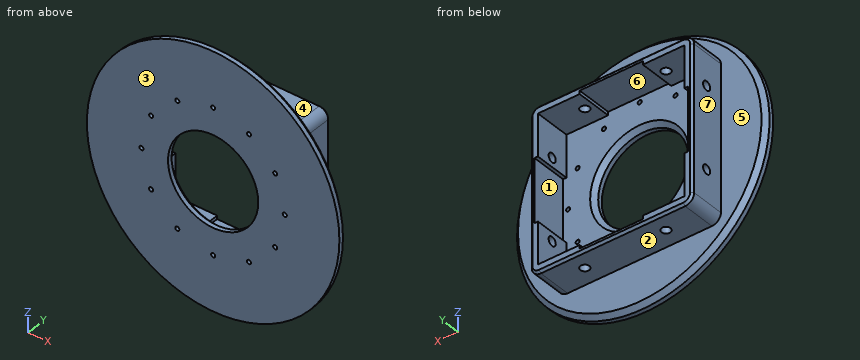
```python
from build123d import *

# Parameters (mm, degrees)
SKETCH1_R               = 88.9
SKETCH1_W               = 114.3
SKETCH1_H               = 114.3
BOSS_EXTRUDE1_DEPTH     = 6.35
SKETCH1_R_2             = 1.4351
SKETCH1_R_3             = 31.75
BOSS_EXTRUDE1_2_DEPTH   = 6.35
SKETCH1_3_W             = 114.3
SKETCH1_3_H             = 114.3
BOSS_EXTRUDE2_DEPTH     = 31.75
SKETCH3_R               = 3.175
CUT_EXTRUDE1_DEPTH      = 89.9
CUT_EXTRUDE1_DEPTH_BACK = 89.9
SKETCH4_R               = 3.175
CUT_EXTRUDE2_DEPTH      = 89.9
CUT_EXTRUDE2_DEPTH_BACK = 89.9
FILLET1_R               = 6.35
CHAMFER1_SIZE           = 3.175
CHAMFER2_SIZE           = 1.5875


with BuildPart() as part:
    # Sketch1 → Boss-Extrude1 (new body)
    with BuildSketch(Plane(origin=(0, 0, 0), x_dir=(1, 0, 0), z_dir=(0, 1, 0))):
        Circle(SKETCH1_R)
        Rectangle(SKETCH1_W, SKETCH1_H, mode=Mode.SUBTRACT)
    extrude(amount=BOSS_EXTRUDE1_DEPTH)



with BuildPart() as body_2:
    # Sketch1 → Boss-Extrude1 2 (new body)
    with BuildSketch(Plane(origin=(0, 0, 0), x_dir=(1, 0, 0), z_dir=(0, 1, 0))):
        Polygon((-22.225, -53.975), (22.225, -53.975), (22.225, -51.59375), (51.59375, -51.59375), (51.59375, -22.225), (53.975, -22.225), (53.975, 22.225), (51.59375, 22.225), (51.59375, 51.59375), (22.225, 51.59375), (22.225, 53.975), (-22.225, 53.975), (-22.225, 51.59375), (-51.59375, 51.59375), (-51.59375, 22.225), (-53.975, 22.225), (-53.975, -22.225), (-51.59375, -22.225), (-51.59375, -51.59375), (-22.225, -51.59375), align=None)
        with Locations((0, 50.4444)):
            Circle(SKETCH1_R_2, mode=Mode.SUBTRACT)
        Circle(SKETCH1_R_3, mode=Mode.SUBTRACT)
        with Locations((25.2222, 43.686131879)):
            Circle(SKETCH1_R_2, mode=Mode.SUBTRACT)
        with Locations((43.686131879, 25.2222)):
            Circle(SKETCH1_R_2, mode=Mode.SUBTRACT)
        with Locations((50.4444, 0)):
            Circle(SKETCH1_R_2, mode=Mode.SUBTRACT)
        with Locations((43.686131879, -25.2222)):
            Circle(SKETCH1_R_2, mode=Mode.SUBTRACT)
        with Locations((25.2222, -43.686131879)):
            Circle(SKETCH1_R_2, mode=Mode.SUBTRACT)
        with Locations((0, -50.4444)):
            Circle(SKETCH1_R_2, mode=Mode.SUBTRACT)
        with Locations((-25.2222, -43.686131879)):
            Circle(SKETCH1_R_2, mode=Mode.SUBTRACT)
        with Locations((-43.686131879, -25.2222)):
            Circle(SKETCH1_R_2, mode=Mode.SUBTRACT)
        with Locations((-50.4444, 0)):
            Circle(SKETCH1_R_2, mode=Mode.SUBTRACT)
        with Locations((-43.686131879, 25.2222)):
            Circle(SKETCH1_R_2, mode=Mode.SUBTRACT)
        with Locations((-25.2222, 43.686131879)):
            Circle(SKETCH1_R_2, mode=Mode.SUBTRACT)
    extrude(amount=BOSS_EXTRUDE1_2_DEPTH)


with BuildPart() as part_1:
    add(part.part)

    add(body_2.part)  # Boss-Extrude2 merges body 2
    # Sketch1<3> → Boss-Extrude2 (add)
    with BuildSketch(Plane(origin=(0, 0, 0), x_dir=(1, 0, 0), z_dir=(0, 1, 0))):
        Rectangle(SKETCH1_3_W, SKETCH1_3_H)
        Polygon((22.225, 53.975), (22.225, 51.59375), (51.59375, 51.59375), (51.59375, 22.225), (53.975, 22.225), (53.975, -22.225), (51.59375, -22.225), (51.59375, -51.59375), (22.225, -51.59375), (22.225, -53.975), (-22.225, -53.975), (-22.225, -51.59375), (-51.59375, -51.59375), (-51.59375, -22.225), (-53.975, -22.225), (-53.975, 22.225), (-51.59375, 22.225), (-51.59375, 51.59375), (-22.225, 51.59375), (-22.225, 53.975), align=None, mode=Mode.SUBTRACT)
    extrude(amount=BOSS_EXTRUDE2_DEPTH)

    # Sketch3 → Cut-Extrude1 (cut, two sides)
    with BuildSketch(Plane.XY) as cut_extrude1_sk:
        with Locations((-28.575, 19.05)):
            Circle(SKETCH3_R)
        with Locations((28.575, 19.05)):
            Circle(SKETCH3_R)
    extrude(amount=CUT_EXTRUDE1_DEPTH, mode=Mode.SUBTRACT)
    extrude(cut_extrude1_sk.sketch, amount=-CUT_EXTRUDE1_DEPTH_BACK, mode=Mode.SUBTRACT)

    # Sketch4 → Cut-Extrude2 (cut, two sides)
    with BuildSketch(Plane(origin=(0, 0, 0), x_dir=(0, 0, -1), z_dir=(1, 0, 0))) as cut_extrude2_sk:
        with Locations((-28.575, 19.05)):
            Circle(SKETCH4_R)
        with Locations((28.575, 19.05)):
            Circle(SKETCH4_R)
    extrude(amount=CUT_EXTRUDE2_DEPTH, mode=Mode.SUBTRACT)
    extrude(cut_extrude2_sk.sketch, amount=-CUT_EXTRUDE2_DEPTH_BACK, mode=Mode.SUBTRACT)

    # Fillet1
    fillet1_edges = [part_1.edges().sort_by_distance(p)[0] for p in [
        (-57.15, 19.05, -57.15),
        (-57.15, 19.05, 57.15),
        (57.15, 19.05, 57.15),
        (57.15, 19.05, -57.15),
    ]]
    fillet(fillet1_edges, radius=FILLET1_R)

    # Chamfer1
    chamfer1_edges = [part_1.edges().sort_by_distance(p)[0] for p in [
        (-88.9, 6.35, 0),
        (-31.75, 6.35, 0),
    ]]
    chamfer(chamfer1_edges, length=CHAMFER1_SIZE)

    # Chamfer2
    chamfer2_edges = [part_1.edges().sort_by_distance(p)[0] for p in [
        (0, 31.75, 57.15),
        (-57.15, 31.75, 0),
        (57.15, 31.75, 0),
        (0, 31.75, -57.15),
        (55.290128061, 31.75, 55.290128061),
        (55.290128061, 31.75, -55.290128061),
        (-55.290128061, 31.75, -55.290128061),
        (-55.290128061, 31.75, 55.290128061),
    ]]
    chamfer(chamfer2_edges, length=CHAMFER2_SIZE)


solid = part_1.part
```
Input: part model. Units: mm. Frame: model coordinates. Face numbers are marked on the shaded views. A direction names the side the tool comes from. Coordinates: 2 decimals unless noted, no trailing zeros. Write each loop counter-clockwise with the first axis right and the second up, starting at its lowest first coordinate (ties: lowest second). Pieces come first, ordered by that corner, then holes. Notation, with made-up numbers: (-11.75, 22.25) - (8.25, 22.25) arc R19 ccw to (8.25, 38.25) - close; hole circle Ø5 at (65, 80.5). An arc over 180 degrees is marked (long way). Put each result on its own line as item: value. Start each with the question number.
1) Contact query for flat-ended pins moving along their axis: pin 1 (1.5 mm diameter, centred on x = -25, z = 51, fed in from -Y); pin 2 (8.5 mm diameter, centred on x = -28.575, y = 19.05, fed in from -Z); pin 3 (19 mm diameter, centred on y = 20, z = -21.5, fed in from -X); pin 4 (2 mm diameter, centred on y = 8, z = 48, fed in from +X). Output: stop coordinate, or through.
2) Reachability of the marked faces 1, 2, 3 and 4 from +Z, -Z, +X, -X, +Y, -Y: full face, straight path, thin tool, end or side. Return the list, or none.
3) Ray query, L1, parallel to Z at x = 0, y = 2.3; L2, parallel to Z at x = 45, y = 10.5. Return the intervals inside material, ascending.
4) Mould query, pull axis X, two halves, no side actions, for the marked faces 5, 6 and 7. Classes: pulls with the +X half, pulls with the -X half, needs draft (parallel to the pull), parting line crosses it, or undercut.
5) Cut plane A-A (y = 26.5). Return the cut outline in (x, z) (3 decimals), plus the area to 3 significant figures.
Resolved:
1. pin 1: stops at y = 0
1. pin 2: stops at z = -57.15
1. pin 3: stops at x = -57.15
1. pin 4: stops at x = 57.15
2. face 1: +Y
2. face 2: -Z, +X, -X, +Y
2. face 3: +Z, -Z, +X, -X, -Y
2. face 4: +Z, +X, -X, +Y
3. L1: z = -88.9 to -51.88, -49.01 to -31.75, 31.75 to 49.01, 51.88 to 88.9
3. L2: z = -57.15 to -51.59, 51.59 to 57.15
4. face 5: needs draft
4. face 6: undercut
4. face 7: pulls with the -X half
5. outline: (-57.15, -50.8) arc R6.35 ccw to (-50.8, -57.15) - (50.8, -57.15) arc R6.35 ccw to (57.15, -50.8) - (57.15, 50.8) arc R6.35 ccw to (50.8, 57.15) - (-50.8, 57.15) arc R6.35 ccw to (-57.15, 50.8) - close; hole (-53.975, -22.225) - (-51.594, -22.225) - (-51.594, -51.594) - (-22.225, -51.594) - (-22.225, -53.975) - (22.225, -53.975) - (22.225, -51.594) - (51.594, -51.594) - (51.594, -22.225) - (53.975, -22.225) - (53.975, 22.225) - (51.594, 22.225) - (51.594, 51.594) - (22.225, 51.594) - (22.225, 53.975) - (-22.225, 53.975) - (-22.225, 51.594) - (-51.594, 51.594) - (-51.594, 22.225) - (-53.975, 22.225) - close
5. area: 1,960 mm2
